Can you work these out from the drawing? Everything is in mm from the part's minimum corner. A direction names the side the tool comes from. Round coordinates to 2 decimals unless told otherwise and drop trailing zeros. Write each loop counter-clockwise with the first axis right and the second up, starting at its lowest first coordinate (ties: lowest second). Pieces come first, ordered by that corner, then holes.
Q1. I'm going to push flat-ended pins straight in: pin 1 Ø4 at (x, y) = (6, 43) entering from +Z; pin 2 Ø1.6 at (y, z) = (51, 14.5) entering from -X; pin 3 Ø1 at (y, z) = (50.5, 16) entering from -X. Where does each tip first touch, or does it pass through?
Q2. We'd pull the mould along Y, two halves only. Please class the marked faces 3, 4, 5 and 6: +Y half, -Y half, draft (parallel to the pull), parting line (faces both ways), or undercut.
Q3. For the marked faces 1 and 2, which set-ups out of +Z, -Z, +X, -X, +Y, -Y let a thin tool reach every point of the face, with its end or its side?
Q4. If we section it at C-C (y = 21.5): Please give me the cut outline in (x, z).
Q5. Please list where these lines run through material, in increasing order: line 1 along Y through (x, z) = (18, 5.5); line 2 along Z through (x, y) = (6.5, 48.5); line 3 along Z through (x, y) = (21.75, 29.5).
Q6. If we section it at B-B (z = 11): Please give me the cut outline in (x, y), plus the area to 3 significant figures.
Q7. If we section it at A-A (x = 9.25): Please give me the cut outline in (y, z), plus the area to 3 significant figures.
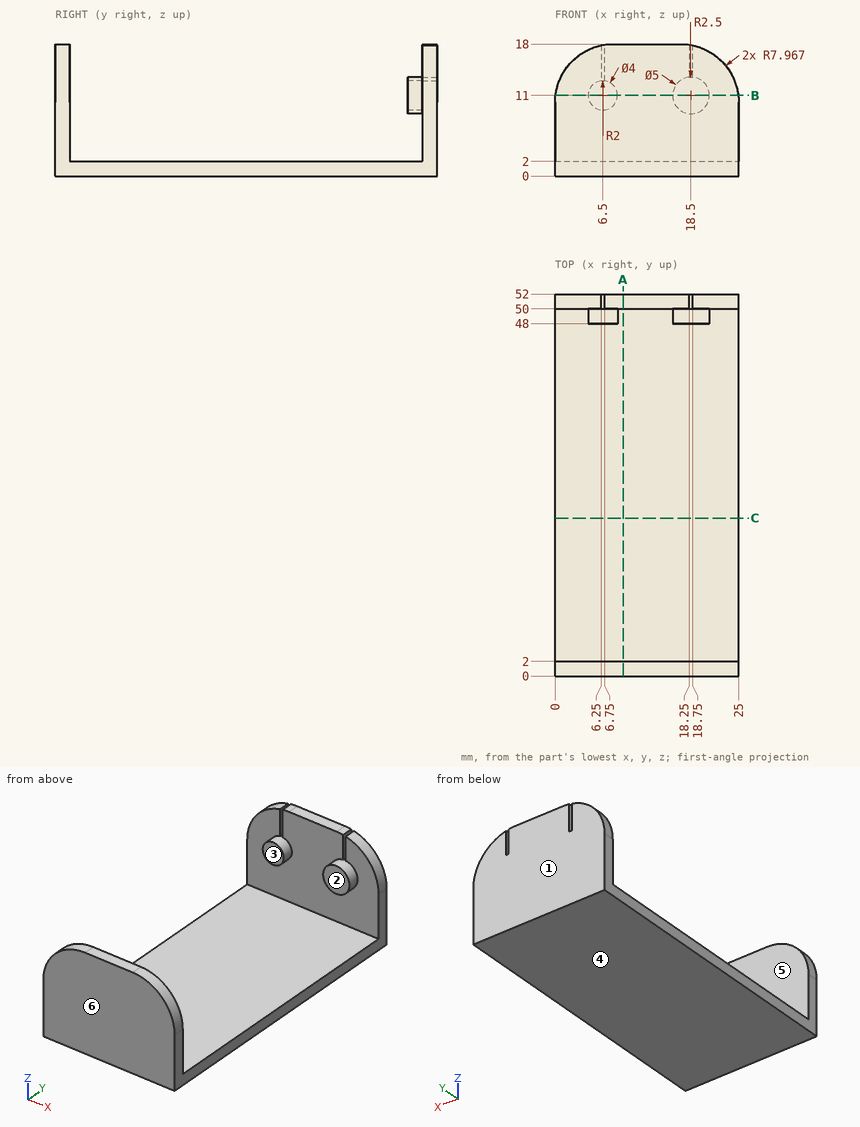
A:
1. pin 1: stops at z = 2
1. pin 2: stops at x = 0.89
1. pin 3: stops at x = 2.17
2. face 3: undercut
2. face 4: draft
2. face 5: undercut
2. face 6: -Y half
3. face 1: +Z, -Z, +X, -X, +Y
3. face 2: +Z, +X, -X
4. outline: (0, 0) - (25, 0) - (25, 2) - (0, 2) - close
5. line 1: y = 0 to 2, 50 to 52
5. line 2: z = 0 to 2, 9 to 13
5. line 3: z = 0 to 2
6. outline: (0.06, 0) - (24.94, 0) - (24.94, 2) - (0.06, 2) - close; (0.06, 50) - (4.5, 50) - (4.5, 48) - (8.5, 48) - (8.5, 50) - (16, 50) - (16, 48) - (21, 48) - (21, 50) - (24.94, 50) - (24.94, 52) - (0.06, 52) - close
6. area: 118 mm2
7. outline: (0, 0) - (52, 0) - (52, 18) - (50, 18) - (50, 2) - (2, 2) - (2, 18) - (0, 18) - close
7. area: 168 mm2
